from build123d import *

# Parameters (mm, degrees)
SKETCH1_R           = 19
BOSS_EXTRUDE2_DEPTH = 15
SKETCH3_R           = 19
CUT_EXTRUDE1_DEPTH  = 56.83030278
BOSS_EXTRUDE3_DEPTH = 3
CIRPATTERN1_COUNT   = 4


with BuildPart() as part:
    # Sketch1 → Boss-Extrude2 (new body)
    with BuildSketch(Plane(origin=(0, 0, 0), x_dir=(1, 0, 0), z_dir=(0, 1, 0))):
        Polygon((21.04758878, 21.04758878), (0, 29.765785508), (-21.04758878, 21.04758878), (-29.765785508, 0), (-21.04758878, -21.04758878), (0, -29.765785508), (21.04758878, -21.04758878), (29.765785508, 0), align=None)
        Circle(SKETCH1_R, mode=Mode.SUBTRACT)
    extrude(amount=BOSS_EXTRUDE2_DEPTH)

    # Sketch2 → Revolve2 (revolve)
    with BuildSketch(Plane.XY):
        with BuildLine():
            Line((26.5, 46.83030278), (26.5, 55.83030278))
            Line((26.5, 55.83030278), (0, 55.83030278))
            Line((0, 55.83030278), (0, 15))
            Line((0, 15), (26.5, 15))
            Line((26.5, 15), (26.5, 28.5))
            ThreePointArc((26.5, 28.5), (20.5, 37.66515139), (26.5, 46.83030278))
        make_face()
    revolve(axis=Axis((0, 102.251774254, 0), (0, -1, 0)))

    # Sketch3 → Cut-Extrude1 (cut, through all)
    with BuildSketch(Plane(origin=(0, 55.83030278, 0), x_dir=(1, 0, 0), z_dir=(0, 1, 0))):
        Circle(SKETCH3_R)
    extrude(amount=-CUT_EXTRUDE1_DEPTH, mode=Mode.SUBTRACT)

    # Sketch4 → Boss-Extrude3 (add, symmetric)
    with BuildSketch(Plane(origin=(0, 7.5, 0), x_dir=(1, 0, 0), z_dir=(0, 1, 0))):
        Polygon((22.145562855, 18.396844877), (28.280721426, 3.585261849), (32.797723404, 13.585261849), align=None)
    boss_extrude3 = extrude(amount=BOSS_EXTRUDE3_DEPTH, both=True)

    # Sketch6 → Cut-Revolve1 (revolve, cut)
    with BuildSketch(Plane.XY):
        Polygon((26.5, 23), (22.169872981, 20.5), (26.5, 18), align=None)
    revolve(axis=Axis((0, -19.954319923, 0), (0, 1, 0)), mode=Mode.SUBTRACT)

    # CirPattern1: Boss-Extrude3 ×4 about axis
    cirpattern1_axis = Axis((0, 0, 0), (0, 1, 0))
    for i in range(1, CIRPATTERN1_COUNT):
        add(boss_extrude3.rotate(cirpattern1_axis, i * 360 / CIRPATTERN1_COUNT))


solid = part.part
Geometry: final body of the model. Coordinates: model frame, mm. A direction names the side the tool comes from. Round coordinates to 2 decimals unless told otherwise and drop trailing zeros. Loops run counter-clockwise (first coordinate to the right, second up) from the corner with the lowest first, then second, coordinate; pieces in that order, holes last. Notation, with made-up numbers: M 25,38 L 82,38 A7 cw 82,43 Z; hole C 57,39 d8. An arc over 180 degrees is marked long. Put each result on its own line as item: value. Start each with the question number.
(1) Section query C-C (y = 44.5). Return loops of the section in (x, z).
(2) Section query A-A (y = 8.5). Return loops of the section in (x, z).
(3) Contact query for flat-ended pins moving along their axis: pin 1 Ø12 at (x, y) = (-10.5, 35.5) entering from +Z; pin 2 Ø3 at (x, z) = (-13.5, -27.5) entering from +Y; pin 3 Ø8 at (x, y) = (13, 31.5) entering from +Z. Output: stop coordinate, or through.
(4) Material intervals for line 1 along Y through (x, z) = (21.5, -13); line 2 along X through (y, z) = (14, 0), sorted ascending. Write a range as [from, to].
(5) Draft query along Z for faces 6 (the face through (-10.376, 4.062, -25.468)), 7 (the face through (-18, 15, -20)), 8 (the face through (-30.5, 7.5, 8.5)), 9 (the face through (14.246, 25.788, 22.345)). Return one class per face: +Z half, -Z half, draft (parallel to the pull), parting line (faces both ways), or undercut.
(6) Set-up query: faces 1 (the face through (-17.76, 20.62, 13.62)), 2 (the face through (30.5, 7.5, -8.5)), 3 (the face through (8.5, 7.5, 30.5)), 4 (the face through (-27, 4.5, 11)), 5 (the face through (27, 4.5, -11)). Return all of +Z, -Z, +X, -X, +Y, -Y with unobstructed straight access to the full face (end or side cutting, diameter ignored); none if empty.
(7) Section query B-B (y = 27). Return loops of the section in (x, z).
Findings below:
1. outline: C 0,0 d46.4; hole C 0,0 d38
2. outline: M -32.8,13.59 L -28.28,3.59 L -29.77,0 L -21.05,-21.05 L -18.4,-22.15 L -13.59,-32.8 L -3.59,-28.28 L 0,-29.77 L 21.05,-21.05 L 22.15,-18.4 L 32.8,-13.59 L 28.28,-3.59 L 29.77,0 L 21.05,21.05 L 18.4,22.15 L 13.59,32.8 L 3.59,28.28 L 0,29.77 L -21.05,21.05 L -22.15,18.4 Z; hole C 0,0 d38
3. pin 1: stops at z = 22.75
3. pin 2: stops at y = 10.5
3. pin 3: stops at z = 24.39
4. line 1: y = [0, 18.79], [22.21, 29.23], [46.1, 55.83]
4. line 2: x = [-29.77, -19], [19, 29.77]
5. face 6: -Z half
5. face 7: draft
5. face 8: undercut
5. face 9: parting line
6. face 1: none
6. face 2: +X, +Y, -Y
6. face 3: +Z, +Y, -Y
6. face 4: +Z, -X, -Y
6. face 5: -Z, +X, -Y
7. outline: C 0,0 d53; hole C 0,0 d38
